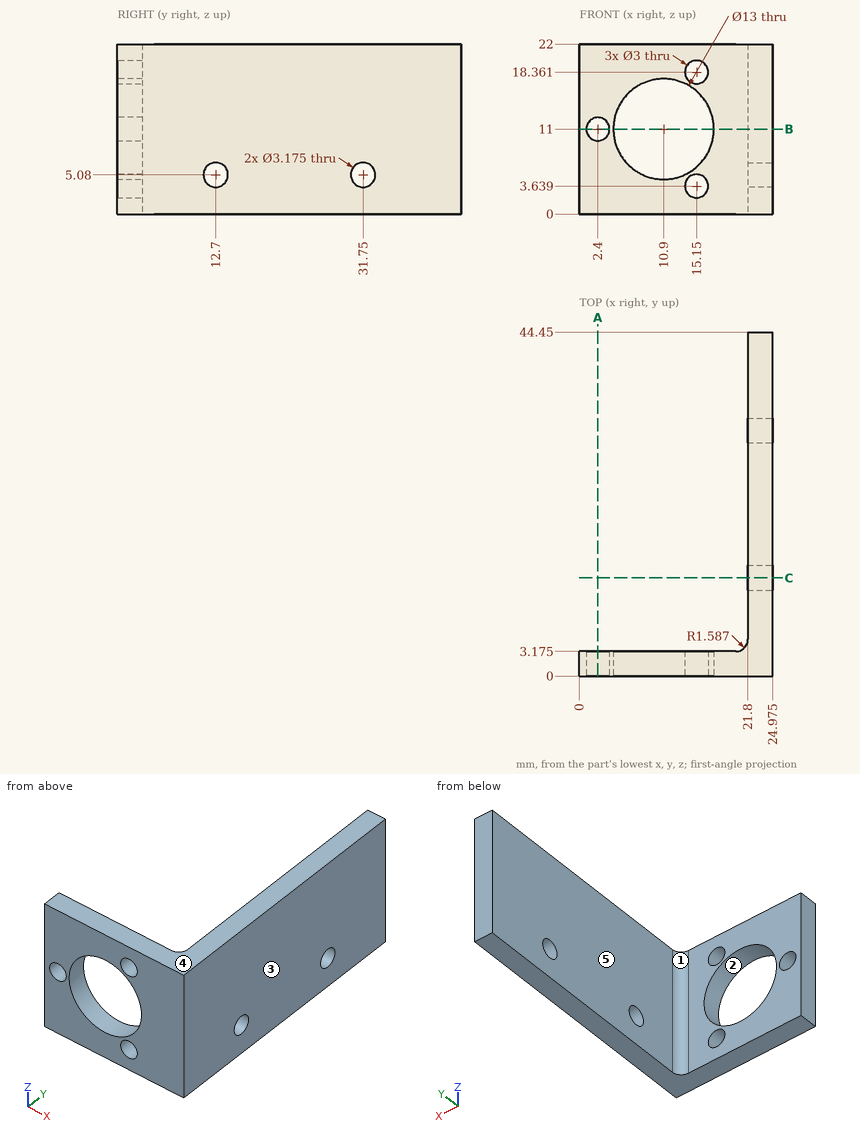
Can you work these out from the drawing? Everything is in mm from the part's minimum corner. A direction names the side the tool comes from. Coordinates: 2 decimals unless noted, no trailing zeros. Loops run counter-clockwise (first coordinate to the right, second up) from the corner with the lowest first, then second, coordinate; pieces in that order, holes last. Notation, with made-up numbers: (-18.75, 29) - (29.25, 29) arc R17 ccw to (29.25, 49) - close; hole circle Ø10 at (82, -31). An arc over 180 degrees is marked (long way). Use a Markdown table: item, result.
Item 1: I want a section at B-B on z = 11. Give the number of separate pieces and of enclosed holes in the cut face, and give its area (3 significant figures).
Numbers:
| item | result |
|---|---|
| separate pieces | 3 |
| enclosed holes | 0 |
| area | 160 mm2 |
Item 2: Will these pins go through, and if not, where does the flat tip stop? pin 1 (3.5 mm diameter, centred on y = 31.75, z = 5.08, fed in from +X) (1 decimal); pin 2 (5 mm diameter, centred on x = 15.15, z = 3.64, fed in from +Y) (1 decimal); pin 3 (6 mm diameter, centred on y = 21, z = 5, fed in from -X).
Numbers:
| item | result |
|---|---|
| pin 1 | stops at x = 25 |
| pin 2 | stops at y = 3.2 |
| pin 3 | stops at x = 21.8 |
Item 3: We'd pull the mould along X, two halves only. Please class the marked faces 1, 2 and 3: released by +X, released by -X, zero draft, split by the parting line, or undercut.
Numbers:
| item | result |
|---|---|
| face 1 | released by -X |
| face 2 | undercut |
| face 3 | released by +X |
Item 4: I want a section at C-C on y = 12.7. Please give me the cut outline in (x, z) (1 decimal).
Numbers:
| item | result |
|---|---|
| outline | (21.8, 0) - (25, 0) - (25, 3.5) - (21.8, 3.5) - close; (21.8, 6.7) - (25, 6.7) - (25, 22) - (21.8, 22) - close |
Item 5: For the marked faces 4 and 5, which set-ups out of +Z, -Z, +X, -X, +Y, -Y let a thin tool reach every point of the face, with its end or its side?
Numbers:
| item | result |
|---|---|
| face 4 | +Z, +X, -X, +Y, -Y |
| face 5 | +Z, -Z, -X, +Y |
Item 6: I want a section at A-A on x = 2.4. Please give me the cut outline in (y, z) (1 decimal).
Numbers:
| item | result |
|---|---|
| outline | (0, 0) - (3.2, 0) - (3.2, 9.5) - (0, 9.5) - close; (0, 12.5) - (3.2, 12.5) - (3.2, 22) - (0, 22) - close |
Item 7: If I drill on probe 1 along Y at (x, z) = (23.1, 5.08); probe 2 along Y at (x, z) = (6, 17.75) (1 decimal); probe 3 along X at (y, z) = (10, 15) (1 decimal), over which ranges is the centre line in solid material (lowest first)? Write a range as from..to.
Numbers:
| item | result |
|---|---|
| probe 1 | y = 0..11.11, 14.29..30.16, 33.34..44.45 |
| probe 2 | y = 0..3.2 |
| probe 3 | x = 21.8..25 |
